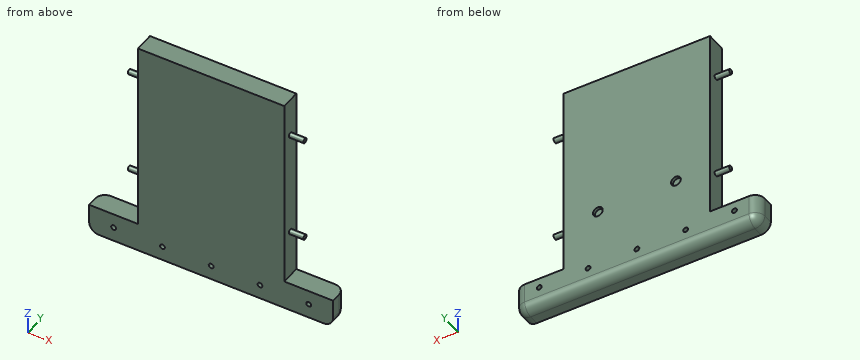
```python
from build123d import *

# Parameters (mm, degrees)
BOSS_EXTRUDE1_DEPTH      = 20
SKETCH4_R                = 2.5
CUT_EXTRUDE2_DEPTH       = 5
FILLET1_R                = 10
FILLET2_R                = 10
SKETCH6_R                = 2.5
CUT_EXTRUDE3_DEPTH       = 5
SKETCH8_R                = 5
CUT_EXTRUDE5_DEPTH       = 3
BOSS_EXTRUDE2_DEPTH      = 15
BOSS_EXTRUDE2_DEPTH_BACK = 165
SKETCH2_R                = 2.5


with BuildPart() as part:
    # Sketch1 → Boss-Extrude1 (new body)
    with BuildSketch(Plane(origin=(0, 0, 0), x_dir=(1, 0, 0), z_dir=(0, 1, 0))):
        Polygon((-75, -100), (75, -100), (75, 100), (125, 100), (125, 130), (-125, 130), (-125, 100), (-75, 100), align=None)
    extrude(amount=BOSS_EXTRUDE1_DEPTH)

    # Sketch4 → Cut-Extrude2 (cut)
    with BuildSketch(Plane.XZ):
        with Locations(Location((-100, -115, 0), (0, 0, 270))):
            Circle(SKETCH4_R)
        with Locations(Location((-50, -115, 0), (0, 0, 270))):
            Circle(SKETCH4_R)
        with Locations(Location((0, -115, 0), (0, 0, 270))):
            Circle(SKETCH4_R)
        with Locations(Location((50, -115, 0), (0, 0, 90))):
            Circle(SKETCH4_R)
        with Locations(Location((100, -115, 0), (0, 0, 90))):
            Circle(SKETCH4_R)
    extrude(amount=-CUT_EXTRUDE2_DEPTH, mode=Mode.SUBTRACT)

    # Fillet1
    fillet1_edges = [part.edges().sort_by_distance(p)[0] for p in [
        (-125, 10, -130),
        (125, 10, -130),
    ]]
    fillet(fillet1_edges, radius=FILLET1_R)

    # Fillet2
    fillet2_edges = [part.edges().sort_by_distance(p)[0] for p in [
        (125, 20, -110),
        (0, 20, -130),
        (-125, 20, -110),
        (-122.071067812, 20, -127.071067812),
        (122.071067812, 20, -127.071067812),
    ]]
    fillet(fillet2_edges, radius=FILLET2_R)

    # Sketch6 → Cut-Extrude3 (cut)
    with BuildSketch(Plane(origin=(0, 20, 0), x_dir=(1, 0, 0), z_dir=(0, 1, 0))):
        with Locations(Location((0, 110, 0), (0, 0, 270))):
            Circle(SKETCH6_R)
        with Locations(Location((50, 110, 0), (0, 0, 270))):
            Circle(SKETCH6_R)
        with Locations(Location((100, 110, 0), (0, 0, 270))):
            Circle(SKETCH6_R)
        with Locations(Location((-50, 110, 0), (0, 0, 90))):
            Circle(SKETCH6_R)
        with Locations(Location((-100, 110, 0), (0, 0, 90))):
            Circle(SKETCH6_R)
    extrude(amount=-CUT_EXTRUDE3_DEPTH, mode=Mode.SUBTRACT)

    # Sketch8 → Cut-Extrude5 (cut)
    with BuildSketch(Plane(origin=(0, 20, 0), x_dir=(1, 0, 0), z_dir=(0, 1, 0))):
        with Locations(Location((-40, 50, 0), (0, 0, 270))):
            Circle(SKETCH8_R)
        with Locations(Location((40, 50, 0), (0, 0, 90))):
            Circle(SKETCH8_R)
    extrude(amount=-CUT_EXTRUDE5_DEPTH, mode=Mode.SUBTRACT)

    # Sketch2 → Boss-Extrude2 (add, two sides: drawn at the far end of the back side and taken through both)
    with BuildSketch(Plane.ZY.offset(75).offset(-BOSS_EXTRUDE2_DEPTH_BACK)):
        with Locations((60, 10)):
            Circle(SKETCH2_R)
        with Locations((-50, 10)):
            Circle(SKETCH2_R)
    extrude(amount=BOSS_EXTRUDE2_DEPTH + BOSS_EXTRUDE2_DEPTH_BACK)


solid = part.part
```
Check sheet for the modelled part. Datum: model origin and axes. Units: mm. Coordinates: 2 decimals unless noted, no trailing zeros. Loops run counter-clockwise (first coordinate to the right, second up) from the corner with the lowest first, then second, coordinate; pieces in that order, holes last. Notation, with made-up numbers: M 76.5,19.25 L 82.5,19.25 A18 cw 82.5,35.25 Z; hole C 23,26 d1. An arc over 180 degrees is marked long. Answer as a JSON object with one key per item and string values.
1. Sectioned sample at B-B on z = -58. Record the cut outline in (x, y), and give its area (3 significant figures).
Outcome:
{"outline": "M -75,0 L 75,0 L 75,20 L -75,20 Z", "area": "3,000 mm²"}
2. Scan lines: L1, parallel to X at y = 3.95, z = -115; L2, parallel to Z at x = -87, y = 9.75; L3, parallel to X at y = 16.2, z = -110. Record each from-to range of solid material in increasing order. Write a range as from..to.
Outcome:
{"L1": "-125..-102.5, -97.5..-52.5, -47.5..-2.5, 2.5..47.5, 52.5..97.5, 102.5..125", "L2": "-130..-100, -52.49..-47.51, 57.51..62.49", "L3": "-122.85..-102.5, -97.5..-52.5, -47.5..-2.5, 2.5..47.5, 52.5..97.5, 102.5..122.85"}
3. Sectioned sample at A-A on x = 107.5. Record the cut outline in (y, z), and give its area (3 significant figures).
Outcome:
{"outline": "M 0,-130 L 10,-130 A10 ccw 20,-120 L 20,-100 L 0,-100 Z", "area": "579 mm²"}
4. Depth check by flat-ended pin: P1, Ø4, axis at y = 10, z = 60, coming from the +X side; P2, Ø3, axis at x = 38, z = -49, coming from the +Y side; P3, Ø1.5, axis at x = 50.5, z = -110.5, coming from the +Y side. Enter the tip coordinate at first touch or a pass-through.
Outcome:
{"P1": "x = 90", "P2": "y = 17", "P3": "y = 15"}
